Can you work these out from the model? Positions are in its coordinate system, mm. A direction names the side the tool comes from. Round coordinates to 2 decimals unless told otherwise and drop trailing zeros. Loops run counter-clockwise (first coordinate to the right, second up) from the corner with the lowest first, then second, coordinate; pieces in that order, holes last.
Autodesk Inventor part; units mm, degrees
ref_plane "YZ Plane" through (0, 0, 0) normal (1, 0, 0) x (0, 1, 0)
ref_plane "XZ Plane" through (0, 0, 0) normal (0, 1, 0) x (-1, 0, 0)
ref_plane "XY Plane" through (0, 0, 0) normal (0, 0, 1) x (1, 0, 0)
sketch "Náčrt1" plane through (0, 0, 0) normal (0, 0, 1) x (1, 0, 0)
  line L0 (-7, 0) -> (7, 0)
  line L1 (0, 9.6) -> (0, -1.6)
  line L2 (-5, 8) -> (-5, 0)
  line L3 (-5, 0) -> (5, 0)
  line L4 (5, 0) -> (5, 8)
  line L5 (5, 8) -> (3.5, 8)
  line L6 (3.5, 8) -> (3.5, 1.5)
  line L7 (3.5, 1.5) -> (-3.5, 1.5)
  line L8 (-3.5, 1.5) -> (-3.5, 8)
  line L9 (-3.5, 8) -> (-5, 8)
  point P0 (0, 0)
  point P1 (-5, 0)
  dimension "d0" = 1.5
  dimension "d1" = 1.5
  dimension "d2" = 1.5
  dimension "d3" = 10
  dimension "d4" = 8
  dimension "d5" = 8
extrude "Vysunutí1" add sketch "Náčrt1" along normal mid plane 42
sketch "Náčrt2" plane through (0, 0, 21) normal (0, 0, 1) x (1, 0, 0)
  line L0 (-5, 8) -> (-5, 0)
  line L1 (-5, 0) -> (5, 0)
  line L2 (5, 0) -> (5, 8)
  line L3 (5, 8) -> (3.5, 8)
  line L4 (3.5, 8) -> (3.5, 1.5)
  line L5 (3.5, 1.5) -> (-3.5, 1.5)
  line L6 (-3.5, 1.5) -> (-3.5, 8)
  line L7 (-3.5, 8) -> (-5, 8)
  line L8 (-5, 0) -> (5, 0)
  line L9 (5, 0) -> (5, 1.5)
  line L10 (5, 1.5) -> (-5, 1.5)
  line L11 (-5, 1.5) -> (-5, 0)
  point P0 (0, 0)
extrude "Vysunutí2" add sketch "Náčrt2" along normal blind 1 contours L10 L5 L2 L1 L0
sketch "Náčrt3" plane through (0, 0, 22) normal (0, 0, 1) x (1, 0, 0)
  line L0 (-5, 1.5) -> (-5, 0)
  line L1 (-5, 0) -> (5, 0)
  line L2 (5, 0) -> (5, 1.5)
  line L3 (5, 1.5) -> (-5, 1.5)
  line L4 (5, 1.5) -> (5, 0)
  line L5 (5, 0) -> (-5, 0)
  line L6 (5, 0) -> (-5, 0)
  line L7 (-5, 0) -> (-5, 1.5)
  line L8 (-5, 1.5) -> (-2.7769, 7.608)
  line L9 (-5, 1.5) -> (1.5, 1.5) construction
  line L10 (-2.7769, 7.608) -> (-1.3673, 7.095)
  line L11 (-1.3673, 7.095) -> (-3.4037, 1.5)
  line L12 (0, 9.6) -> (0, -1.6)
  line L13 (5, 1.5) -> (2.7769, 7.608)
  line L14 (2.7769, 7.608) -> (1.3673, 7.095)
  line L15 (1.3673, 7.095) -> (3.4037, 1.5)
  line L16 (-3.4037, 1.5) -> (3.4037, 1.5)
  point P0 (0, 0)
  dimension "d10" = 6.5
  dimension "d11" = 70
  dimension "d12" = 1.5
extrude "Vysunutí3" add sketch "Náčrt3" along normal blind 2
fillet "Zaoblení1" radius 0.75 8 edges at (-5, 8, 0) (-3.5, 8, 0) (3.5, 8, 0) (5, 8, 0) (1.3673, 7.095, 23) (2.7769, 7.608, 23) (-2.7769, 7.608, 23) (-1.3673, 7.095, 23)
sketch "Náčrt4" plane through (5, 0, 24) normal (1, 0, 0) x (0, 0, -1)
  line L0 (3, 7.25) -> (45, 7.25)
  line L1 (3, 1.5) -> (3, 7.25)
  line L2 (3, 1.5) -> (2, 1.5)
  line L3 (2, 1.5) -> (0, 1.5)
  line L4 (0, 0) -> (0, 1.5)
  line L5 (45, 0) -> (0, 0)
  line L6 (45, 7.25) -> (45, 0)
  point P0 (24, 0)
  point P1 (9, 2.75)
  point P2 (39, 2.75)
  dimension "d16" = 2.75
  dimension "d17" = 2.75
  dimension "d18" = 6
  dimension "d19" = 30
hole "Díra1" at (5, 2.75, 15) at (5, 2.75, -15) direction (-1, 0, 0) diameter 2.5 end through all
sketch "Náčrt5" plane through (-3.5, 1.5, -21) normal (0, 1, 0) x (1, 0, 0)
  line L0 (7, 0) -> (7, -6)
  line L1 (0, 0) -> (7, 0)
  line L2 (0, 0) -> (0, -6)
  line L3 (0, -6) -> (0, -36)
  line L4 (0, -36) -> (0, -42)
  line L5 (-1.5, -42) -> (0, -42)
  line L6 (-1.5, -42) -> (-1.5, -43)
  line L7 (0.0963, -43) -> (-1.5, -43)
  line L8 (0.0963, -43) -> (0.0963, -45)
  line L9 (6.9037, -45) -> (0.0963, -45)
  line L10 (6.9037, -43) -> (6.9037, -45)
  line L11 (8.5, -43) -> (6.9037, -43)
  line L12 (8.5, -42) -> (8.5, -43)
  line L13 (7, -42) -> (8.5, -42)
  line L14 (7, -36) -> (7, -42)
  line L15 (7, -6) -> (7, -36)
  line L16 (10.5, -21) -> (-3.5, -21)
  line L17 (3.5, 9) -> (3.5, -54)
  point P0 (3.5, -21)
  point P1 (3.5, -12)
  point P2 (3.5, -30)
  dimension "d27" = 12
  dimension "d28" = 18
hole "Díra2" at (0, 1.5, -9) at (0, 1.5, 9) direction (0, -1, 0) diameter 3.2 end through all
properties part number "x_holder" material "Hliník 6061"
(1) If we mould it in two halves opening along Y, with no side actions, what happens to faces 1 (the flat face through (0, 1, 24)), 2 (the flat face through (-4.03, 4.16, 22.99)), 3 (the cylindrical face through (1.65, 6.97, 23.01))? For each: released by +Y, released by -Y, zero draft, split by the parting line, or undercut.
Worked answers:
face 1: zero draft
face 2: released by +Y
face 3: undercut
(2) If we section it at B-B, the plane x = 0: List the corners of the cut face in (y, z) for me, then the cut area to 3 significant figures.
Worked answers:
outline: (0, -21) - (1.5, -21) - (1.5, -10.6) - (0, -10.6) - close; (0, -7.4) - (1.5, -7.4) - (1.5, 7.4) - (0, 7.4) - close; (0, 10.6) - (1.5, 10.6) - (1.5, 24) - (0, 24) - close
area: 57.9 mm2
(3) If we section it at C-C, the plane z = 14.5: State how many separate pieces and enclosed holes the cut face has, then the cut area to 3 significant figures.
Worked answers:
separate pieces: 3
enclosed holes: 0
area: 27.1 mm2
(4) For faces 4 (the flat face through (3.5, 4, 0)), 5 (the flat face through (-5, 4, 1)), 6 (the cylindrical face through (-1.645, 6.956, 23.014)), 7 (the flat face through (3, 4, 22)), which set-ups out of +Z, -Z, +X, -X, +Y, -Y let a thin tool reach every point of the face, with its end or its side?
Worked answers:
face 4: -Z, +Y
face 5: +Z, -Z, -X, +Y, -Y
face 6: +Z, -Z
face 7: +X, -X, +Y
(5) Will these pins go through, and if not, where does the flat tip stop? P1, Ø3, axis at x = 1.5, z = 0, coming from the +Y side; P2, Ø0.8, axis at x = -4, y = 6, coming from the +Z side; P3, Ø1.5, axis at y = 2.75, z = 15, coming from the -X side; P4, Ø1.7, axis at x = 2.5, y = 4, coming from the -Z side.
Worked answers:
P1: stops at y = 1.5
P2: stops at z = 21
P3: passes through
P4: stops at z = 22
(6) If I drill on line 1 (Z direction, x = -4, y = 2.75); line 2 (Z direction, x = 0, y = 0.45); line 3 (Z direction, x = 4.6, y = 2.75), over which ranges is the centre line in solid material (lowest first)?
Worked answers:
line 1: z = -21 to -16.25, -13.75 to 13.75, 16.25 to 21, 22 to 24
line 2: z = -21 to -10.6, -7.4 to 7.4, 10.6 to 24
line 3: z = -21 to -16.25, -13.75 to 13.75, 16.25 to 21
